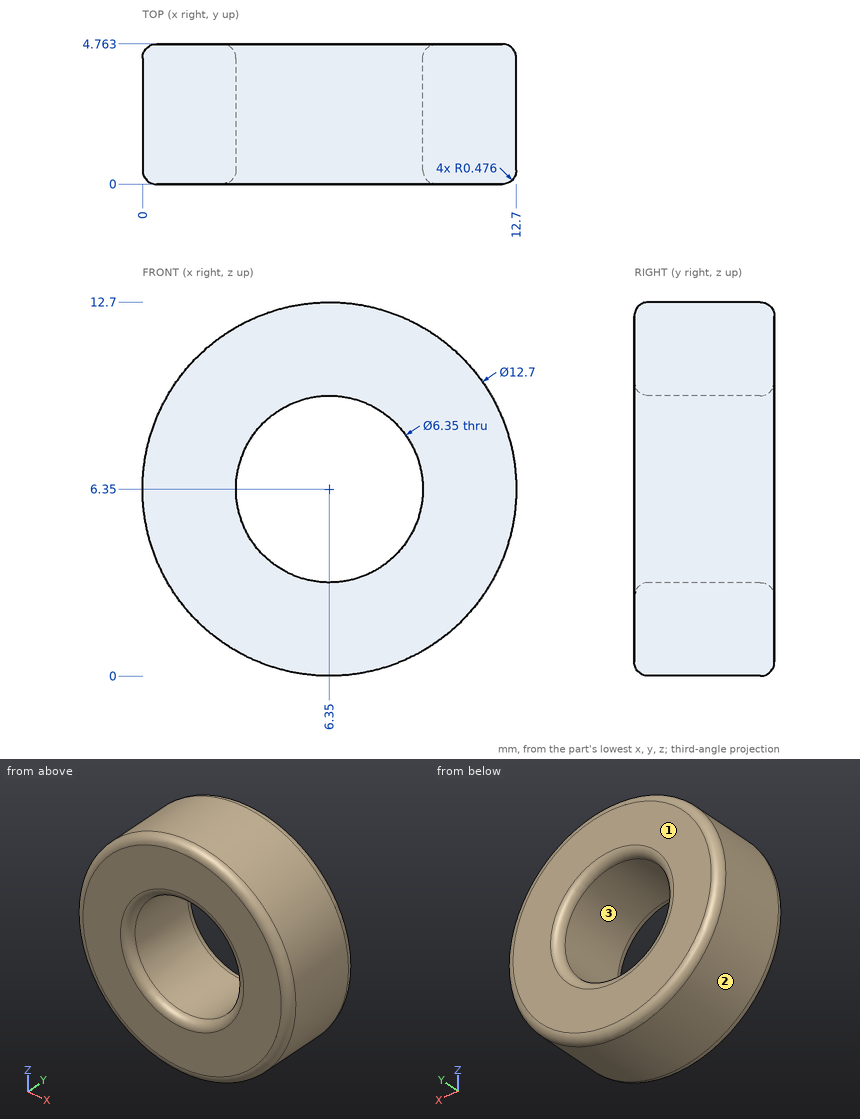
Can you work these out from the drawing? Everything is in mm from the part's minimum corner. Round coordinates to 2 decimals unless told otherwise and drop trailing zeros. Write item = value, one per line.
1. Thinking about a two-plate mould opening in X: for the marked faces 1, 2 and 3, which applies, +X half, -X half, draft (parallel to the pull), parting line (faces both ways), or undercut?
Results below:
face_1 = draft
face_2 = parting line
face_3 = undercut
2. Will these pins go through, and if not, where does the flat tip stop? P1, Ø1, axis at y = 2.5, z = 2, coming from the -X side; P2, Ø2, axis at y = 1, z = 3.5, coming from the -X side (1 decimal); P3, Ø1, axis at y = 3, z = 7, coming from the -X side.
Results below:
P1 = 1.3
P2 = 0.3
P3 = 0
3. I need wall thicknesses on probe 1 along Z at (x, y) = (6.35, 3.3) (1 decimal); probe 2 along Z at (x, y) = (5.5, 2.4); probe 3 along X at (y, z) = (3.7, 9) (1 decimal). Which ranges of each line are inside material? Lowest first, please.
Results below:
probe_1 = 0 to 3.2, 9.5 to 12.7
probe_2 = 0.06 to 3.29, 9.41 to 12.64
probe_3 = 0.6 to 4.6, 8.1 to 12.1
